Build history of the part. All positions in model axes, mm. Face numbers are marked on the shaded views. A direction names the side the tool comes from. Round coordinates to 2 decimals unless told otherwise and drop trailing zeros. Write each loop counter-clockwise with the first axis right and the second up, starting at its lowest first coordinate (ties: lowest second). Pieces come first, ordered by that corner, then holes. Notation, with made-up numbers: (4, 6) -> (29, 6) arc R13 ccw to (29, 30) -> close; hole circle Ø7 at (-16.75, -27.75). An arc over 180 degrees is marked (long way). Answer in a Markdown table with one row per item.
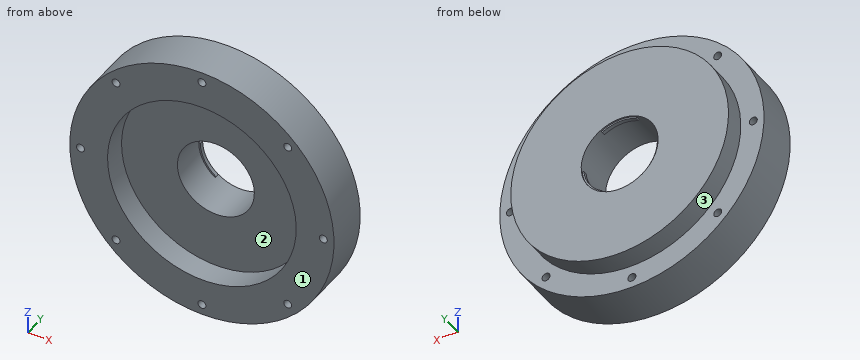
```python
from build123d import *

# Parameters (mm, degrees)
SKETCH1_R                = 91
SKETCH1_R_2              = 65
SKETCH1_R_3              = 2.75
BOSS_EXTRUDE1_DEPTH      = 30
BOSS_EXTRUDE2_DEPTH      = 14
BOSS_EXTRUDE2_DEPTH_BACK = 14
SKETCH2_R                = 75
SKETCH2_R_2              = 26.5
SKETCH5_W                = 1.1
SKETCH5_H                = 2.6
REVOLVE1_ANGLE           = 55
CIRPATTERN1_COUNT        = 3


with BuildPart() as part:
    # Sketch1 → Boss-Extrude1 (new body)
    with BuildSketch(Plane(origin=(0, 0, 0), x_dir=(1, 0, 0), z_dir=(0, 1, 0))):
        with Locations(Location((0, 0, 0), (0, 0, 270))):
            Circle(SKETCH1_R)
        with Locations(Location((0, 0, 0), (0, 0, 270))):
            Circle(SKETCH1_R_2, mode=Mode.SUBTRACT)
        with Locations(Location((0, 83.635, 0), (0, 0, 270))):
            Circle(SKETCH1_R_3, mode=Mode.SUBTRACT)
        with Locations(Location((59.138875645, 59.138875645, 0), (0, 0, 270))):
            Circle(SKETCH1_R_3, mode=Mode.SUBTRACT)
        with Locations(Location((83.635, 0, 0), (0, 0, 270))):
            Circle(SKETCH1_R_3, mode=Mode.SUBTRACT)
        with Locations(Location((59.138875645, -59.138875645, 0), (0, 0, 270))):
            Circle(SKETCH1_R_3, mode=Mode.SUBTRACT)
        with Locations(Location((0, -83.635, 0), (0, 0, 270))):
            Circle(SKETCH1_R_3, mode=Mode.SUBTRACT)
        with Locations(Location((-59.138875645, -59.138875645, 0), (0, 0, 270))):
            Circle(SKETCH1_R_3, mode=Mode.SUBTRACT)
        with Locations(Location((-83.635, 0, 0), (0, 0, 270))):
            Circle(SKETCH1_R_3, mode=Mode.SUBTRACT)
        with Locations(Location((-59.138875645, 59.138875645, 0), (0, 0, 270))):
            Circle(SKETCH1_R_3, mode=Mode.SUBTRACT)
    extrude(amount=BOSS_EXTRUDE1_DEPTH)

    # Sketch2 → Boss-Extrude2 (add, two sides: drawn at the far end of the back side and taken through both)
    with BuildSketch(Plane(origin=(0, 30, 0), x_dir=(1, 0, 0), z_dir=(0, 1, 0)).offset(-BOSS_EXTRUDE2_DEPTH_BACK)):
        with Locations(Location((0, 0, 0), (0, 0, 270))):
            Circle(SKETCH2_R)
        with Locations(Location((0, 0, 0), (0, 0, 270))):
            Circle(SKETCH2_R_2, mode=Mode.SUBTRACT)
    extrude(amount=BOSS_EXTRUDE2_DEPTH + BOSS_EXTRUDE2_DEPTH_BACK)

    # Sketch5 → Revolve1 (revolve)
    with BuildSketch(Plane.XY):
        with Locations((-25.95, 41.7)):
            Rectangle(SKETCH5_W, SKETCH5_H)
    revolve1 = revolve(axis=Axis((0, 48.211759647, 0), (0, -1, 0)), revolution_arc=REVOLVE1_ANGLE)

    # CirPattern1: Revolve1 ×3 about axis
    cirpattern1_axis = Axis((0, 0, 0), (0, 1, 0))
    for i in range(1, CIRPATTERN1_COUNT):
        add(revolve1.rotate(cirpattern1_axis, i * 360 / CIRPATTERN1_COUNT))


solid = part.part
```
Q1. Drop flat-ended pins along their axis: P1, Ø9, axis at x = 59.14, z = -59.14, coming from the +Y side; P2, Ø3.5, axis at x = -1.5, z = 25, coming from the -Y side; P3, Ø2, axis at y = 39, z = 46, coming from the +X side; P4, Ø3.5, axis at x = 59.14, z = 59.14, coming from the -Y side. Give the stop position or say it passes through.
A:
| item | result |
|---|---|
| P1 | y = 30 |
| P2 | y = 16 |
| P3 | x = 60 |
| P4 | through |
Q2. Saw through at A-A on x = 0. Write the cut outline in (y, z) (3 decimals).
A:
| item | result |
|---|---|
| outline | (0, -91) -> (30, -91) -> (30, -86.385) -> (0, -86.385) -> close; (0, -80.885) -> (30, -80.885) -> (30, -75) -> (44, -75) -> (44, -26.5) -> (16, -26.5) -> (16, -65) -> (0, -65) -> close; (0, 65) -> (16, 65) -> (16, 26.5) -> (40.4, 26.5) -> (40.4, 25.4) -> (43, 25.4) -> (43, 26.5) -> (44, 26.5) -> (44, 75) -> (30, 75) -> (30, 80.885) -> (0, 80.885) -> close; (0, 86.385) -> (30, 86.385) -> (30, 91) -> (0, 91) -> close |
Q3. Wall check: line 1 (X direction, y = 18, z = 0) (3 decimals); line 2 (X direction, y = 8, z = 0) (3 decimals); line 3 (Y direction, x = 5, z = -48.5). Give the ranges that are in metal, low to high. Write a range as [from, to].
A:
| item | result |
|---|---|
| line 1 | [-91, -86.385], [-80.885, -26.5], [26.5, 80.885], [86.385, 91] |
| line 2 | [-91, -86.385], [-80.885, -65], [65, 80.885], [86.385, 91] |
| line 3 | [16, 44] |
Q4. Which spindle directions (+Z, -Z, +X, -X, +Y, -Y) get a long thin tool onto all of the face, cutting with end or side? Do the marked faces 1, 2 and 3. Say none if no direction does.
A:
| item | result |
|---|---|
| face 1 | +Z, -Z, +X, -X, -Y |
| face 2 | -Y |
| face 3 | +Y |
Q5. Saw through at C-C on x = 53.5. Write the cut outline in (y, z).
A:
| item | result |
|---|---|
| outline | (0, -73.61) -> (30, -73.61) -> (30, -52.56) -> (44, -52.56) -> (44, 52.56) -> (30, 52.56) -> (30, 73.61) -> (0, 73.61) -> (0, 36.92) -> (16, 36.92) -> (16, -36.92) -> (0, -36.92) -> close |
Q6. Saw through at D-D on x = -31. Write the cut outline in (y, z).
A:
| item | result |
|---|---|
| outline | (0, -85.56) -> (30, -85.56) -> (30, -68.29) -> (44, -68.29) -> (44, 68.29) -> (30, 68.29) -> (30, 85.56) -> (0, 85.56) -> (0, 57.13) -> (16, 57.13) -> (16, -57.13) -> (0, -57.13) -> close |
Q7. Saw through at B-B on y = 3. State how many separate pieces and enclosed holes the cut face has, plus the area to 3 significant figures.
A:
| item | result |
|---|---|
| separate pieces | 1 |
| enclosed holes | 9 |
| area | 12,600 mm² |
